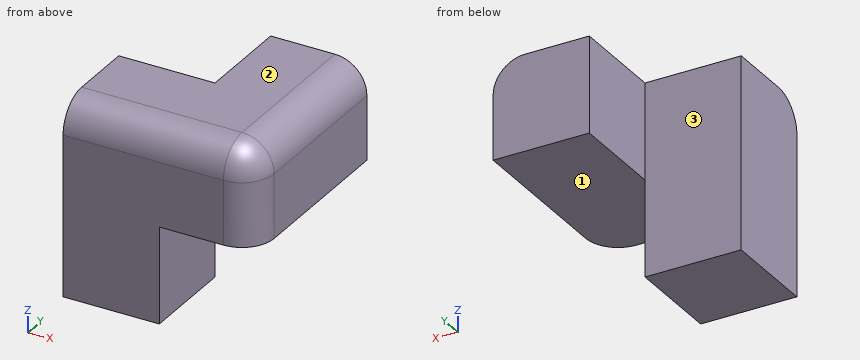
```python
from build123d import *

# Parameters (mm, degrees)
F1_DEPTH = 38.1
F2_W     = 19.05
F2_H     = 19.05
F3_DEPTH = 38.101
F4_R     = 6.35
F5_R     = 6.35


with BuildPart() as f1:
    # F0 (on Front) → F1 (new body)
    with BuildSketch(Plane.XZ):
        Polygon((0, 35.814), (0, -2.286), (19.05, -2.286), (19.05, 16.764), (38.1, 16.764), (38.1, 35.814), align=None)
    extrude(amount=F1_DEPTH)

    # F2 (on face) → F3 (cut, through all)
    with BuildSketch(Plane.XY.offset(35.814)):
        with Locations((9.525, -9.525)):
            Rectangle(F2_W, F2_H)
    extrude(amount=-F3_DEPTH, mode=Mode.SUBTRACT)

    # F4
    f4_edges = [f1.edges().sort_by_distance(p)[0] for p in [
        (19.05, -38.1, 35.814),
    ]]
    fillet(f4_edges, radius=F4_R)

    # F5
    f5_edges = [f1.edges().sort_by_distance(p)[0] for p in [
        (38.1, -15.875, 35.814),
    ]]
    fillet(f5_edges, radius=F5_R)


solid = f1.part
```
The listing builds one solid part. Answer for the finished solid, in the listing's coordinates (mm). Face numbers are marked on the shaded views. A direction names the side the tool comes from. Give positions to 0.01 mm unless a question says otherwise; leave off trailing zeros. Order: outer loops, then holes, each group sorted by start corner. A loop starts at its lowest first (then second) coordinate and runs counter-clockwise, first axis right, second up. Notation, with made-up numbers: (26, -23.75) - (43, -23.75) arc R16 cw to (43, 2.25) - close; hole circle Ø6 at (53, 78.5). An arc over 180 degrees is marked (long way). Answer in a Markdown table with one row per item. Add a question column.
Q1. The part is cut by section D-D (y = -4). Determine the outline of the cut face in (x, z).
Q2. The part is cut by section B-B (y = -28). Determine the outline of the cut face in (x, z), then the cut area to 3 significant figures.
Q3. Given P1, Ø2, axis at x = 15.5, z = 5, coming from the +Y side; P2, Ø5.5, axis at y = -11, z = 30.5, coming from the -X side; P3, Ø21, axis at x = 30.5, y = -14.5, coming from the -Z side, each flat-ended and moving along its own axis, determine where each tip first touches the part or whether it passes through.
Q4. Find the intervals of material crossed by line 1 along Z through (x, y) = (27.5, -8); line 2 along Y through (x, z) = (10.5, 5); line 3 along X through (y, z) = (-20.5, 1), in increasing order. Write a range as [from, to].
Q5. The part is cut by section C-C (x = 15). Determine the outline of the cut face in (y, z), then the cut area to 3 significant figures.
Q6. The part is cut by section A-A (z = 20.5). Determine the outline of the cut face in (x, y).
Q7. Which of the six approach directions +Z, -Z, +X, -X, +Y, -Y give full straight-line access (tool end or side, diameter ignored) to the marked faces 1, 2 and 3?
Determined:
| question | item | result |
|---|---|---|
| 1 | outline | (19.05, 16.76) - (38.1, 16.76) - (38.1, 29.46) arc R6.35 ccw to (31.75, 35.81) - (19.05, 35.81) - close |
| 2 | outline | (0, -2.29) - (19.05, -2.29) - (19.05, 16.76) - (38.1, 16.76) - (38.1, 29.46) arc R6.35 ccw to (31.75, 35.81) - (0, 35.81) - close |
| 2 | area | 1,080 mm² |
| 3 | P1 | stops at y = -19.05 |
| 3 | P2 | stops at x = 19.05 |
| 3 | P3 | stops at z = 16.76 |
| 4 | line 1 | z = [16.76, 35.81] |
| 4 | line 2 | y = [-38.1, -19.05] |
| 4 | line 3 | x = [0, 19.05] |
| 5 | outline | (-38.1, -2.29) - (-19.05, -2.29) - (-19.05, 35.81) - (-31.75, 35.81) arc R6.35 ccw to (-38.1, 29.46) - close |
| 5 | area | 717 mm² |
| 6 | outline | (0, -38.1) - (31.75, -38.1) arc R6.35 ccw to (38.1, -31.75) - (38.1, 0) - (19.05, 0) - (19.05, -19.05) - (0, -19.05) - close |
| 7 | face 1 | -Z, +X, +Y, -Y |
| 7 | face 2 | +Z, +X, -X, +Y, -Y |
| 7 | face 3 | +Z, -Z, -X, +Y |
